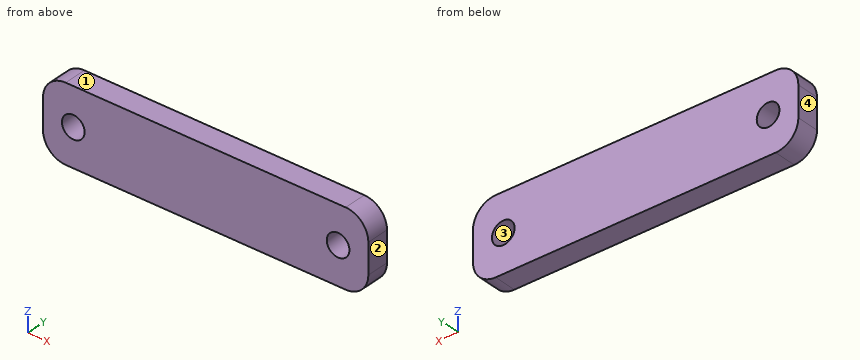
from build123d import *

# Parameters (mm, degrees)
SKETCH1_W             = 43
SKETCH1_H             = 10
BOSS_EXTRUDE1_DEPTH   = 3
FILLET1_R             = 3
F_3_0MM_DOWEL_HOLE1_D = 3


with BuildPart() as part:
    # Sketch1 → Boss-Extrude1 (new body)
    with BuildSketch(Plane(origin=(0, 0, 0), x_dir=(1, 0, 0), z_dir=(0, 1, 0))):
        Rectangle(SKETCH1_W, SKETCH1_H)
    extrude(amount=BOSS_EXTRUDE1_DEPTH)

    # Fillet1
    fillet1_edges = [part.edges().sort_by_distance(p)[0] for p in [
        (21.5, 1.5, 5),
        (-21.5, 1.5, 5),
        (-21.5, 1.5, -5),
        (21.5, 1.5, -5),
    ]]
    fillet(fillet1_edges, radius=FILLET1_R)

    # Ø3.0mm Dowel Hole1 (through all)
    with Locations(Plane(origin=(0, 0, 0), x_dir=(-1, 0, 0), z_dir=(0, -1, 0))):
        with Locations((-17.5, 0), (17.5, 0)):
            Hole(F_3_0MM_DOWEL_HOLE1_D / 2)


solid = part.part
Read the model definition and answer for the solid it produces. Units are mm, in the model's axes. Face numbers are marked on the shaded views. Give positions to 0.01 mm unless a question says otherwise; leave off trailing zeros. Write each loop counter-clockwise with the first axis right and the second up, starting at its lowest first coordinate (ties: lowest second). Pieces come first, ordered by that corner, then holes. Notation, with made-up numbers: M 78,33 L 98,33 A18 ccw 98,60 Z; hole C 15,18.5 d11. An arc over 180 degrees is marked long. One line per item, written item: value. Start each with the question number.
(1) Find the intervals of material crossed by line 1 (Z direction, x = 17.5, y = 2.15); line 2 (X direction, y = 0.5, z = 0.75); line 3 (Z direction, x = 17, y = 2.6), in increasing order.
(2) Find section C-C (x = 17.5). Determine the outline of the cut face in (y, z).
(3) Determine the mould class of the marked faces 1, 2, 3 and 4 for opening direction X: pulls with the +X half, pulls with the -X half, needs draft (parallel to the pull), parting line crosses it, or undercut.
(4) Find section B-B (y = 2.4). Determine the outline of the cut face in (x, z).
(5) Find section D-D (z = 4). Determine the outline of the cut face in (x, y), plus the area to 3 significant figures.
(6) Find section A-A (z = 0). Determine the outline of the cut face in (x, y).
Results below:
1. line 1: z = -5 to -1.5, 1.5 to 5
1. line 2: x = -21.5 to -18.8, -16.2 to 16.2, 18.8 to 21.5
1. line 3: z = -5 to -1.41, 1.41 to 5
2. outline: M 0,-5 L 3,-5 L 3,-1.5 L 0,-1.5 Z; M 0,1.5 L 3,1.5 L 3,5 L 0,5 Z
3. face 1: needs draft
3. face 2: pulls with the +X half
3. face 3: undercut
3. face 4: pulls with the -X half
4. outline: M -21.5,-2 A3 ccw -18.5,-5 L 18.5,-5 A3 ccw 21.5,-2 L 21.5,2 A3 ccw 18.5,5 L -18.5,5 A3 ccw -21.5,2 Z; hole C -17.5,0 d3; hole C 17.5,0 d3
5. outline: M -20.74,0 L 20.74,0 L 20.74,3 L -20.74,3 Z
5. area: 124 mm^2
6. outline: M -21.5,0 L -19,0 L -19,3 L -21.5,3 Z; M -16,0 L 16,0 L 16,3 L -16,3 Z; M 19,0 L 21.5,0 L 21.5,3 L 19,3 Z
